```python
from build123d import *

# Parameters (mm, degrees)
SKETCH1_W           = 76.155927022
SKETCH1_H           = 76.155927022
SKETCH1_R           = 9.525
BOSS_EXTRUDE1_DEPTH = 25.4
SKETCH2_W           = 12.7
SKETCH2_H           = 6.35
CUT_EXTRUDE1_DEPTH  = 89.852780068


with BuildPart() as part:
    # Sketch1 → Boss-Extrude1 (new body)
    with BuildSketch(Plane(origin=(0, 0, 0), x_dir=(1, 0, 0), z_dir=(0, 1, 0))):
        Rectangle(SKETCH1_W, SKETCH1_H)
        with Locations(Location((-12.677963511, 12.677963511, 0), (0, 0, 270))):
            Circle(SKETCH1_R, mode=Mode.SUBTRACT)
    extrude(amount=BOSS_EXTRUDE1_DEPTH)

    # Sketch2 → Cut-Extrude1 (cut, through all)
    with BuildSketch(Plane.XY.offset(38.077963511)):
        with Locations((19.139376005, 22.225)):
            Rectangle(SKETCH2_W, SKETCH2_H)
    extrude(amount=-CUT_EXTRUDE1_DEPTH, mode=Mode.SUBTRACT)


solid = part.part
```
Model file for the job. Use its own axes, mm. A direction names the side the tool comes from. Coordinates: 2 decimals unless noted, no trailing zeros. Loops run counter-clockwise (first coordinate to the right, second up) from the corner with the lowest first, then second, coordinate; pieces in that order, holes last. Notation, with made-up numbers: (59.5, 0) -> (117.5, 0) arc R32 ccw to (117.5, 35) -> close; hole circle Ø1 at (32, 50). An arc over 180 degrees is marked (long way). Answer as a JSON object with one key per item and string values.
Q1. Cut at C-C (x = -7.5). List the corners of the cut face in (y, z).
Report:
{"outline": "(0, -38.08) -> (25.4, -38.08) -> (25.4, -20.67) -> (0, -20.67) -> close; (0, -4.68) -> (25.4, -4.68) -> (25.4, 38.08) -> (0, 38.08) -> close"}
Q2. Probe probe 1 along X at (y, z) = (21, -31); probe 2 along X at (y, z) = (5.25, -17.5); probe 3 along Z at (x, y) = (-13.5, 17). List the from-to ranges inside material, lowest first.
Report:
{"probe 1": "x = -38.08 to 12.79, 25.49 to 38.08", "probe 2": "x = -38.08 to -20.89, -4.46 to 38.08", "probe 3": "z = -38.08 to -22.17, -3.19 to 38.08"}
Q3. Cut at B-B (y = 2.5). List the corners of the cut face in (x, z) (3 decimals), and give its area (3 significant figures).
Report:
{"outline": "(-38.078, -38.078) -> (38.078, -38.078) -> (38.078, 38.078) -> (-38.078, 38.078) -> close; hole circle Ø19.05 at (-12.678, -12.678)", "area": "5,510 mm2"}
Q4. Pull direction Z, two halves, no side cores. Call faces 3 (the flat face through (12.789, 22, 1)), 4 (the cylindrical face through (-6.24, 12.52, -19.7)), 5 (the flat face through (-1, 13, -38.078)): released by +Z, released by -Z, zero draft, split by the parting line, or undercut.
Report:
{"face 3": "zero draft", "face 4": "undercut", "face 5": "released by -Z"}
Q5. Cut at D-D (z = -15.5). List the corners of the cut face in (x, y).
Report:
{"outline": "(-38.08, 0) -> (-21.78, 0) -> (-21.78, 25.4) -> (-38.08, 25.4) -> close; (-3.58, 0) -> (38.08, 0) -> (38.08, 25.4) -> (25.49, 25.4) -> (25.49, 19.05) -> (12.79, 19.05) -> (12.79, 25.4) -> (-3.58, 25.4) -> close"}
Q6. Cut at A-A (z = 5.5). List the corners of the cut face in (x, y), and give its area (3 significant figures).
Report:
{"outline": "(-38.08, 0) -> (38.08, 0) -> (38.08, 25.4) -> (25.49, 25.4) -> (25.49, 19.05) -> (12.79, 19.05) -> (12.79, 25.4) -> (-38.08, 25.4) -> close", "area": "1,850 mm2"}
Q7. Flat gauge pins, fed straight in: P1, Ø17, axis at x = -12.68, z = -12.68, coming from the +Y side; P2, Ø14, axis at x = 21, z = -1.5, coming from the +Y side. Where does each tip first touch, or does it go through?
Report:
{"P1": "passes through", "P2": "stops at y = 25.4"}
Q8. 3-axis set-ups, long thin cutter, end or side, ignore diameter. For faces 1 (the flat face through (25.489, 22, 1)), 2 (the flat face through (38.078, 13, 1)): which of +Z, -Z, +X, -X, +Y, -Y reach the whole face in a straight line?
Report:
{"face 1": "+Z, -Z, +Y", "face 2": "+Z, -Z, +X, +Y, -Y"}
